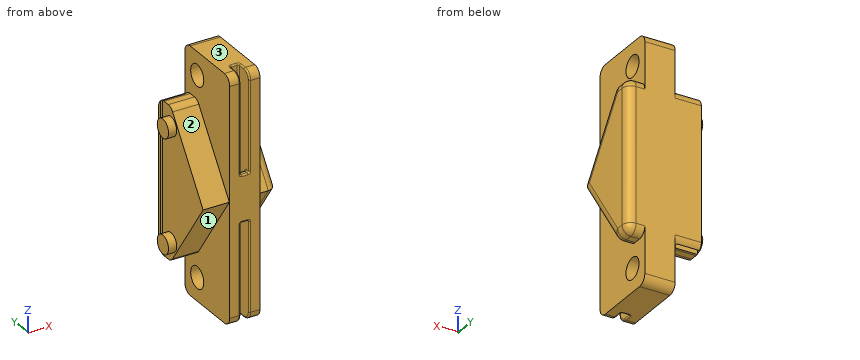
from build123d import *

# Parameters (mm, degrees)
BOSS_EXTRUDE1_DEPTH     = 12.7
SKETCH7_W               = 13
SKETCH7_H               = 0.65
CUT_EXTRUDE2_DEPTH      = 4
SKETCH7_4_R             = 1.6
BOSS_EXTRUDE2_DEPTH     = 1.4
CUT_EXTRUDE3_DEPTH      = 4.5
SKETCH7_6_R             = 1.85
CUT_EXTRUDE4_DEPTH      = 2.4
CUT_EXTRUDE4_DEPTH_BACK = 13.7
CUT_EXTRUDE5_DEPTH      = 3
SKETCH12_W              = 1.5
SKETCH12_H              = 21.000689182
CUT_EXTRUDE6_DEPTH      = 3
SKETCH14_W              = 5.2
SKETCH14_H              = 4
BOSS_EXTRUDE3_DEPTH     = 1
FILLET3_R               = 1.5
FILLET4_R               = 0.25


with BuildPart() as part:
    # Sketch1 → Boss-Extrude1 (new body)
    with BuildSketch(Plane(origin=(0, 0, 0), x_dir=(1, 0, 0), z_dir=(0, 1, 0))):
        Polygon((-28.77817965, 15.54419618), (-24.27817965, 15.54419618), (-24.27817965, 23.54419618), (-19.07817965, 23.54419618), (-19.07817965, 15.54419618), (-16.07817965, 15.54419618), (-16.07817965, 2.54419618), (-28.77817965, 2.54419618), align=None)
    extrude(amount=BOSS_EXTRUDE1_DEPTH)

    # Sketch7 → Cut-Extrude2 (cut)
    with BuildSketch(Plane.ZY.offset(28.77817965)):
        with Locations((-9.04419618, 11.875)):
            Rectangle(SKETCH7_W, SKETCH7_H)
    extrude(amount=-CUT_EXTRUDE2_DEPTH, mode=Mode.SUBTRACT)

    # Sketch7<4> → Boss-Extrude2 (add)
    with BuildSketch(Plane.ZY.offset(28.77817965)):
        with Locations((-12.29419618, 9.2)):
            Circle(SKETCH7_4_R)
    extrude(amount=BOSS_EXTRUDE2_DEPTH)

    # Sketch7<5> → Cut-Extrude3 (cut)
    with BuildSketch(Plane.ZY.offset(28.77817965)):
        Polygon((-2.54419618, 0.097302003), (-15.54419618, 9.2), (-15.54419618, 0), (-2.54419618, 0), align=None)
    extrude(amount=-CUT_EXTRUDE3_DEPTH, mode=Mode.SUBTRACT)

    # Sketch7<6> → Cut-Extrude4 (cut, two sides)
    with BuildSketch(Plane.ZY.offset(28.77817965)) as cut_extrude4_sk:
        with Locations((-19.54419618, 9.2)):
            Circle(SKETCH7_6_R)
    extrude(amount=CUT_EXTRUDE4_DEPTH, mode=Mode.SUBTRACT)
    extrude(cut_extrude4_sk.sketch, amount=-CUT_EXTRUDE4_DEPTH_BACK, mode=Mode.SUBTRACT)

    # Sketch10 → Cut-Extrude5 (cut)
    with BuildSketch(Plane(origin=(-19.07817965, 0, 0), x_dir=(0, 0, -1), z_dir=(1, 0, 0))):
        Polygon((15.54419618, 9.2), (15.54419618, 0), (2.54419618, 0), (2.54419618, 0.097302003), align=None)
    extrude(amount=CUT_EXTRUDE5_DEPTH, mode=Mode.SUBTRACT)

    # Sketch12 → Cut-Extrude6 (cut)
    with BuildSketch(Plane.XZ):
        with Locations((-21.67817965, -13.043851589)):
            Rectangle(SKETCH12_W, SKETCH12_H)
    extrude(amount=-CUT_EXTRUDE6_DEPTH, mode=Mode.SUBTRACT)

    # Sketch14 → Boss-Extrude3 (add)
    with BuildSketch(Plane(origin=(0, 0, 0), x_dir=(-1, 0, 0), z_dir=(0, -1, 0))):
        with Locations((21.67817965, 4.54419618)):
            Rectangle(SKETCH14_W, SKETCH14_H)
    extrude(amount=-BOSS_EXTRUDE3_DEPTH)

    # Fillet3
    fillet3_edges = [part.edges().sort_by_distance(p)[0] for p in [
        (-26.52817965, 9.2, -15.54419618),
        (-17.57817965, 9.2, -15.54419618),
        (-26.52817965, 12.7, -15.54419618),
        (-17.57817965, 12.7, -15.54419618),
        (-16.07817965, 4.648651002, -9.04419618),
        (-16.07817965, 10.95, -15.54419618),
        (-16.07817965, 12.7, -9.04419618),
        (-21.67817965, 12.7, -23.54419618),
        (-23.35317965, 0, -23.54419618),
        (-20.00317965, 0, -23.54419618),
    ]]
    fillet(fillet3_edges, radius=FILLET3_R)

    # Mirror3: part across plane


with BuildPart() as part_1:
    add(part.part)
    add(part.part.mirror(Plane(origin=(-16.07817965, 12.7, -2.54419618), x_dir=(1, 0, 0), z_dir=(0, 0, -1))))

    # Fillet4
    fillet4_edges = [part_1.edges().sort_by_distance(p)[0] for p in [
        (-22.42817965, 0, -14.29419618),
        (-22.42817965, 1, -2.54419618),
        (-22.42817965, 0.5, -6.54419618),
        (-21.67817965, 1, -6.54419618),
        (-20.92817965, 0.5, -6.54419618),
        (-20.92817965, 1, -2.54419618),
        (-21.67817965, 0, -6.54419618),
        (-20.92817965, 0, -14.29419618),
        (-22.42817965, 0.439339828, -23.104856352),
        (-20.92817965, 0.439339828, -23.104856352),
        (-24.77817965, 11.55, -2.54419618),
        (-21.67817965, 3, 18.45580382),
        (-20.92817965, 2.25, 18.45580382),
        (-20.92817965, 0, 9.20580382),
        (-22.42817965, 0, 9.20580382),
        (-22.42817965, 2.25, 18.45580382),
        (-20.92817965, 0.5, 1.45580382),
        (-22.42817965, 0.5, 1.45580382),
        (-21.67817965, 0, 1.45580382),
        (-21.67817965, 1, 1.45580382),
        (-22.42817965, 0.439339828, 18.016463992),
        (-20.92817965, 0.439339828, 18.016463992),
        (-24.77817965, 12.2, -2.54419618),
        (-20.92817965, 3, -2.54419618),
        (-22.42817965, 3, -2.54419618),
        (-22.42817965, 2.25, -23.54419618),
        (-21.67817965, 3, -23.54419618),
        (-20.92817965, 2.25, -23.54419618),
    ]]
    fillet(fillet4_edges, radius=FILLET4_R)


solid = part_1.part
Verification items for the finished model (mm, model axes). Face numbers are marked on the shaded views. A direction names the side the tool comes from. Give positions to 0.01 mm unless a question says otherwise; leave off trailing zeros. Loops run counter-clockwise (first coordinate to the right, second up) from the corner with the lowest first, then second, coordinate; pieces in that order, holes last. Notation, with made-up numbers: (62.25, 75.25) - (107.25, 75.25) arc R27 cw to (107.25, 95.25) - close; hole circle Ø9 at (-32.75, 48). An arc over 180 degrees is marked (long way). Write item = value, one per line. Start each with the question number.
Q1. Cross-section at D-D, the plane y = 9.2. State how many separate pieces and enclosed holes the cut face has, and give its area (3 significant figures).
Q2. Tool access check on the marked faces 1, 2 and 3. Record the directions out of +Z, -Z, +X, -X, +Y, -Y that give a thin tool (end or side, any length) a straight path to the whole face; none if there is none.
Q3. Cross-section at C-C, the plane z = 15.5. Enter the section's corners in (x, y), and give its area (3 significant figures).
Q4. Cross-section at A-A, the plane x = -23.75. Enter the section's corners in (y, z), and give its area (3 significant figures).
Q5. Thickness scan on line 1 (Z direction, x = -20.75, y = 8); line 2 (X direction, y = 7, z = -20); line 3 (X direction, y = 2, z = 7). Record the ranges inside material, lowest first.
Q6. Depth check by flat-ended pin: P1, Ø2, axis at y = 9.2, z = -19.54, coming from the +X side; P2, Ø0.6, axis at x = -22, y = 0.5, coming from the +Z side; P3, Ø5, axis at x = -26.5, z = 8, coming from the -Y side; P4, Ø2, axis at y = 1, z = -4.5, coming from the -X side. Enter the tip coordinate at first touch or a pass-through.
Q7. Cross-section at B-B, the plane x = -26. Enter the section's corners in (y, z), and give its area (3 significant figures).
Answer key:
q1.separate_pieces = 3
q1.enclosed_holes = 0
q1.area = 379 mm^2
q2.face_1 = -Z, -X, -Y
q2.face_2 = +Z, -X, -Y
q2.face_3 = +Z, +X, -X, +Y, -Y
q3.outline = (-24.28, 0) - (-22.68, 0) arc R0.25 ccw to (-22.43, 0.25) - (-22.43, 2.75) arc R0.25 cw to (-22.18, 3) - (-21.18, 3) arc R0.25 cw to (-20.93, 2.75) - (-20.93, 0.25) arc R0.25 ccw to (-20.68, 0) - (-19.08, 0) - (-19.08, 7.67) - (-24.28, 7.67) - close; (-24.28, 10.73) - (-19.08, 10.73) - (-19.08, 12.7) - (-24.28, 12.7) - close
q3.area = 45.7 mm^2
q4.outline = (0, -22.04) arc R1.5 ccw to (1.5, -23.54) - (11.2, -23.54) arc R1.5 ccw to (12.7, -22.04) - (12.7, 16.96) arc R1.5 ccw to (11.2, 18.46) - (1.5, 18.46) arc R1.5 ccw to (0, 16.96) - close; hole circle Ø3.7 at (9.2, -19.54); hole circle Ø3.7 at (9.2, 14.46)
q4.area = 510 mm^2
q5.line_1 = -23.54 to -20.95, -18.14 to 13.05, 15.86 to 18.46
q5.line_2 = -24.28 to -19.08
q5.line_3 = -24.28 to -22.43, -20.93 to -19.08
q6.P1 = through
q6.P2 = 1.49
q6.P3 = 0
q6.P4 = -28.78
q7.outline = (0.1, -2.54) - (8.75, -14.9) arc R1.5 ccw to (9.98, -15.54) - (11.2, -15.54) arc R1.5 ccw to (11.55, -15.5) - (11.55, 10.41) arc R1.5 ccw to (11.2, 10.46) - (9.98, 10.46) arc R1.5 ccw to (8.75, 9.82) - close; (12.2, -15.16) arc R1.5 ccw to (12.7, -14.04) - (12.7, 8.96) arc R1.5 ccw to (12.2, 10.07) - close
q7.area = 192 mm^2
